```python
from build123d import *

# Parameters (mm, degrees)
SKETCH051_R     = 2.7
PAD043_DEPTH    = 11
FILLET001_R     = 0.5
SKETCH050_R     = 1.1
POCKET005_DEPTH = 11


with BuildPart() as part:
    # Sketch051 (on Face1 of CopyFillet) → Pad043 (new body)
    with BuildSketch(Plane.XZ.offset(13)):
        Circle(SKETCH051_R)
    extrude(amount=PAD043_DEPTH)

    # Fillet001
    fillet001_edges = [part.edges().sort_by_distance(p)[0] for p in [
        (-2.7, -24, 0),
    ]]
    fillet(fillet001_edges, radius=FILLET001_R)

    # Sketch050 (on Face4 of Fillet001) → Pocket005 (cut)
    with BuildSketch(Plane.XZ.offset(24)):
        Circle(SKETCH050_R)
    extrude(amount=-POCKET005_DEPTH, mode=Mode.SUBTRACT)


solid = part.part
```
Build history of the part. All positions in model axes, mm. Round coordinates to 2 decimals unless told otherwise and drop trailing zeros. Write each loop counter-clockwise with the first axis right and the second up, starting at its lowest first coordinate (ties: lowest second). Pieces come first, ordered by that corner, then holes. Notation, with made-up numbers: (-21.75, 22) -> (20.25, 22) arc R27 ccw to (20.25, 53) -> close; hole circle Ø7 at (-34, 48). An arc over 180 degrees is marked (long way). Put each result on its own line as item: value.
Item 1: Slice it at B-B, the plane x = 0. Give the cut face in (y, z).
Here are the results:
outline: (-24, -2.2) arc R0.5 ccw to (-23.5, -2.7) -> (-13, -2.7) -> (-13, -1.1) -> (-24, -1.1) -> close; (-24, 1.1) -> (-13, 1.1) -> (-13, 2.7) -> (-23.5, 2.7) arc R0.5 ccw to (-24, 2.2) -> close
Item 2: Two-plate mould, pull along X, no slides. Class faces 1 (the face through (1.05, -18.58, 0.33)), 2 (the face through (-0.585, -18.176, -2.636)), 3 (the face through (-1, -24, 1)): pulls with the +X half, pulls with the -X half, needs draft (parallel to the pull), parting line crosses it, or undercut.
Here are the results:
face 1: undercut
face 2: parting line crosses it
face 3: needs draft
Item 3: Slice it at A-A, the plane z = 0. Give the cut face in (x, y).
Here are the results:
outline: (-2.7, -23.5) arc R0.5 ccw to (-2.2, -24) -> (-1.1, -24) -> (-1.1, -13) -> (-2.7, -13) -> close; (1.1, -24) -> (2.2, -24) arc R0.5 ccw to (2.7, -23.5) -> (2.7, -13) -> (1.1, -13) -> close
Item 4: Wall check: probe 1 along Z at (x, y) = (0, -18.25); probe 2 along X at (y, z) = (-14.75, 0.55). Give the ranges that are in metal, low to high. Write a range as from..to.
Here are the results:
probe 1: z = -2.7..-1.1, 1.1..2.7
probe 2: x = -2.64..-0.95, 0.95..2.64
Item 5: Slice it at C-C, the plane y = -16.75. Give the cut face in (x, z).
Here are the results:
outline: circle Ø5.4 at (0, 0); hole circle Ø2.2 at (0, 0)
Item 6: Flat gauge pin, fed straight in: P1, Ø1, axis at y = -19.5, z = -1.5, coming from the -X side. Where does the tip first touch, or does it go through?
Here are the results:
P1: stops at x = -2.51
